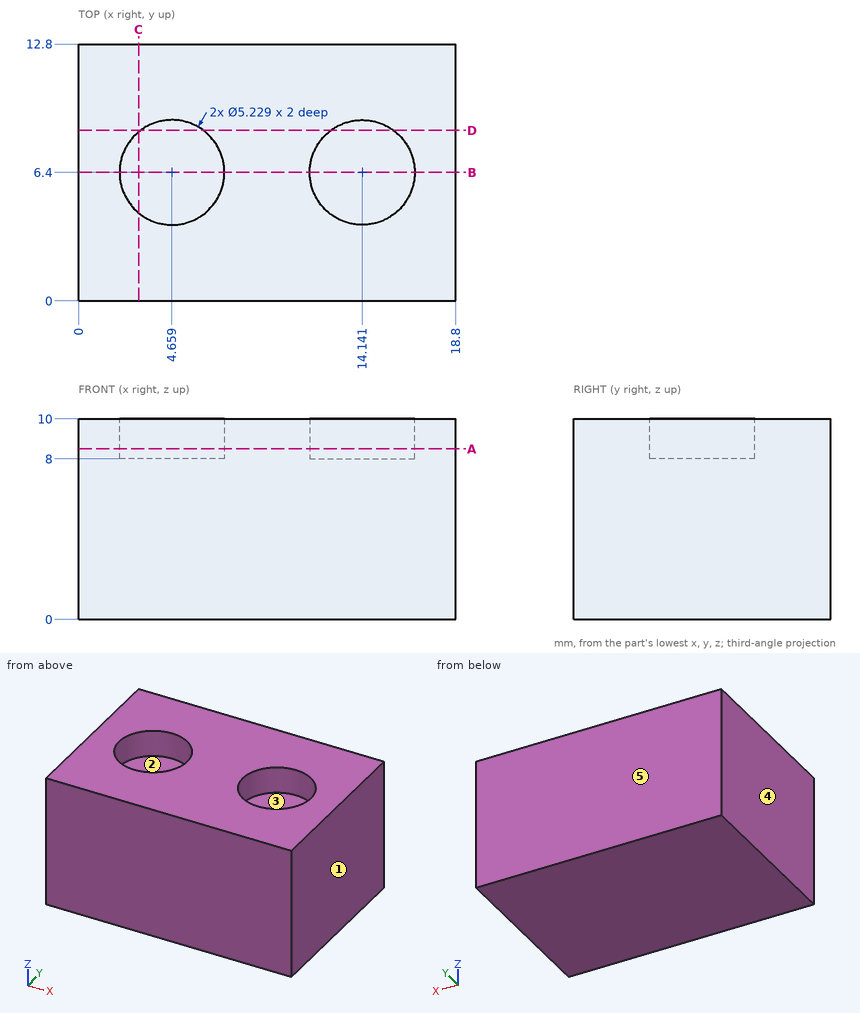
The drawing under review shows one solid part. Ordinate dimensions are in mm from its lowest x, y, z. A direction names the side the tool comes from. Coordinates: 2 decimals unless noted, no trailing zeros. Order: outer loops, then holes, each group sorted by start corner. A loop starts at its lowest first (then second) coordinate and runs counter-clockwise, first axis right, second up. Notation, with made-up numbers: (39.25, 24) - (56.25, 24) arc R19 cw to (56.25, 48) - close; hole circle Ø5 at (-15.5, 13.25). An arc over 180 degrees is marked (long way). Put each result on its own line as item: value.
1) Take a section at B-B, the plane y = 6.4. Give the boundary of the cut face in (x, z) (1 decimal), and give its area (3 significant figures).
Response values:
outline: (0, 0) - (18.8, 0) - (18.8, 10) - (16.8, 10) - (16.8, 8) - (11.5, 8) - (11.5, 10) - (7.3, 10) - (7.3, 8) - (2, 8) - (2, 10) - (0, 10) - close
area: 167 mm²
2) Wall thickness on L1, parallel to X at y = 8, z = 9.25; L2, parallel to Y at x = 4.5, z = 8.25; L3, parallel to Z at x = 2.25, y = 5.5: over which ranges is each line inside the solid? List them lowest first. Write a range as from..to.
Response values:
L1: x = 0..2.59, 6.73..12.07, 16.21..18.8
L2: y = 0..3.79, 9.01..12.8
L3: z = 0..8
3) Take a section at D-D, the plane y = 8.5. Give the boundary of the cut face in (x, z).
Response values:
outline: (0, 0) - (18.8, 0) - (18.8, 10) - (15.7, 10) - (15.7, 8) - (12.58, 8) - (12.58, 10) - (6.22, 10) - (6.22, 8) - (3.1, 8) - (3.1, 10) - (0, 10) - close
4) Tool access review of the marked faces 1 and 2: name each direction out of +Z, -Z, +X, -X, +Y, -Y from which nothing blocks a thin tool from reaching the whole face with its end or side.
Response values:
face 1: +Z, -Z, +X, +Y, -Y
face 2: +Z
5) Take a section at C-C, the plane x = 3. Give the boundary of the cut face in (y, z), and give its area (3 significant figures).
Response values:
outline: (0, 0) - (12.8, 0) - (12.8, 10) - (8.42, 10) - (8.42, 8) - (4.38, 8) - (4.38, 10) - (0, 10) - close
area: 120 mm²
6) Insertion check: P1, Ø4, axis at x = 14.14, y = 6.4, coming from the +Z side. The pin has a flat end and moves straight along its axis. Give the tip position at first contact, or say it passes through.
Response values:
P1: stops at z = 8
7) Take a section at A-A, the plane z = 8.5. Give the boundary of the cut face in (x, y) (1 decimal), and give its area (3 significant figures).
Response values:
outline: (0, 0) - (18.8, 0) - (18.8, 12.8) - (0, 12.8) - close; hole circle Ø5.2 at (4.7, 6.4); hole circle Ø5.2 at (14.1, 6.4)
area: 198 mm²
8) The part is to be moulded in two halves that separate along X. For the marked faces 3, 4 and 5, say which applies: released by +X, released by -X, zero draft, split by the parting line, or undercut.
Response values:
face 3: undercut
face 4: released by -X
face 5: zero draft
